Here's how the part is built. I have some questions about the finished solid (model axes, mm). A direction names the side the tool comes from. Round coordinates to 2 decimals unless told otherwise and drop trailing zeros. Order: outer loops, then holes, each group sorted by start corner. A loop starts at its lowest first (then second) coordinate and runs counter-clockwise, first axis right, second up. Notation, with made-up numbers: (52.25, 8) - (96.25, 8) arc R32 ccw to (96.25, 38) - close; hole circle Ø1 at (48, 32). An arc over 180 degrees is marked (long way). One line per item, written item: value.
from build123d import *
from OCP.BRepFilletAPI import BRepFilletAPI_MakeChamfer

# Parameters (mm, degrees)
SZKIC1_W                    = 50
SZKIC1_H                    = 20
DODANIE_WYCI_GNI_CIE1_DEPTH = 5
SZKIC2_W                    = 20
SZKIC2_H                    = 20
DODANIE_WYCI_GNI_CIE2_DEPTH = 20
SZKIC3_R                    = 2.5
WYTNIJ_WYCI_GNI_CIE1_DEPTH  = 60.371710435
ZAOKR_GLENIE1_R             = 10
SZKIC4_W                    = 50
SZKIC4_H                    = 5
DODANIE_WYCI_GNI_CIE3_DEPTH = 40
SFAZOWANIE1_SIZE            = 10
SFAZOWANIE1_SIZE2           = 37.320508076
SFAZOWANIE2_OUTLINE_R       = 2.5
SFAZOWANIE2_DEPTH           = 20
SFAZOWANIE2_START           = 30
SFAZOWANIE2_2_OUTLINE_R     = 2.5
SFAZOWANIE2_2_DEPTH         = 20
SZKIC5_R                    = 3.043345969
WYTNIJ_WYCI_GNI_CIE2_DEPTH  = 83.006097334


with BuildPart() as part:
    # Szkic1 → Dodanie-wyciągnięcie1 (new body)
    with BuildSketch(Plane.XY):
        with Locations((25, 10)):
            Rectangle(SZKIC1_W, SZKIC1_H)
    extrude(amount=DODANIE_WYCI_GNI_CIE1_DEPTH)

    # Szkic2 → Dodanie-wyciągnięcie2 (add)
    with BuildSketch(Plane.XY.offset(5)):
        with Locations((10, 10)):
            Rectangle(SZKIC2_W, SZKIC2_H)
        with Locations((40, 10)):
            Rectangle(SZKIC2_W, SZKIC2_H)
    extrude(amount=DODANIE_WYCI_GNI_CIE2_DEPTH)

    # Szkic3 → Wytnij-wyciągnięcie1 (cut, through all)
    with BuildSketch(Plane.ZY):
        with Locations((15, 10)):
            Circle(SZKIC3_R)
    extrude(amount=-WYTNIJ_WYCI_GNI_CIE1_DEPTH, mode=Mode.SUBTRACT)

    # Zaokrąglenie1
    zaokr_glenie1_edges = [part.edges().sort_by_distance(p)[0] for p in [
        (40, 20, 25),
        (40, 0, 25),
        (10, 0, 25),
        (10, 20, 25),
    ]]
    fillet(zaokr_glenie1_edges, radius=ZAOKR_GLENIE1_R - 0.0001)  # a hair under: the kernel refuses the full size

    # Szkic4 → Dodanie-wyciągnięcie3 (add)
    with BuildSketch(Plane(origin=(0, 20, 0), x_dir=(1, 0, 0), z_dir=(0, 1, 0))):
        with Locations((25, -2.5)):
            Rectangle(SZKIC4_W, SZKIC4_H)
    extrude(amount=DODANIE_WYCI_GNI_CIE3_DEPTH)

    # Sfazowanie1: one chamfer whose edges measure the first distance from different faces: ONE call of the kernel's chamfer builder (chamfer() names one face for all edges)
    sfazowanie1_edges_1 = [part.edges().sort_by_distance(p)[0] for p in [
        (40, 20, 5),
    ]]
    sfazowanie1_side_1 = [part.faces().sort_by_distance(p)[0] for p in [
        (40, 20, 10.00005),
    ]]
    sfazowanie1_edges_2 = [part.edges().sort_by_distance(p)[0] for p in [
        (10, 20, 5),
    ]]
    sfazowanie1_side_2 = [part.faces().sort_by_distance(p)[0] for p in [
        (10, 20, 10.00005),
    ]]
    sfazowanie1 = BRepFilletAPI_MakeChamfer(part.part.solid().wrapped)
    for e in sfazowanie1_edges_1:
        sfazowanie1.Add(SFAZOWANIE1_SIZE, SFAZOWANIE1_SIZE2, e.wrapped, sfazowanie1_side_1[0].wrapped)  # the first distance lies on this face
    for e in sfazowanie1_edges_2:
        sfazowanie1.Add(SFAZOWANIE1_SIZE, SFAZOWANIE1_SIZE2, e.wrapped, sfazowanie1_side_2[0].wrapped)  # the first distance lies on this face
    add(Compound.cast(sfazowanie1.Shape()), mode=Mode.REPLACE)

    # Sfazowanie2: read off the stored shape, not the designer's step
    # Sfazowanie2 outline → Sfazowanie2 (add)
    with BuildSketch(Plane.YZ):
        with BuildLine():
            Line((0, 15), (0, 0))
            Line((0, 0), (60, 0))
            Line((60, 0), (60, 5))
            Line((60, 5), (57.320508076, 5))
            Line((57.320508076, 5), (31.081570656, 12.030702092))
            Line((31.081570656, 12.030702092), (18.642014143, 20.031460181))
            ThreePointArc((18.642014143, 20.031460181), (7.394250725, 24.654536276), (0, 15))
        make_face()
        with Locations((10, 15)):
            Circle(SFAZOWANIE2_OUTLINE_R, mode=Mode.SUBTRACT)
    extrude(amount=SFAZOWANIE2_DEPTH)

    # Sfazowanie2 2 outline → Sfazowanie2 2 (add)
    with BuildSketch(Plane.YZ.offset(SFAZOWANIE2_START)):
        with BuildLine():
            Line((0, 15), (0, 0))
            Line((0, 0), (60, 0))
            Line((60, 0), (60, 5))
            Line((60, 5), (57.320508076, 5))
            Line((57.320508076, 5), (31.081570656, 12.030702092))
            Line((31.081570656, 12.030702092), (18.642014143, 20.031460181))
            ThreePointArc((18.642014143, 20.031460181), (7.394250725, 24.654536276), (0, 15))
        make_face()
        with Locations((10, 15)):
            Circle(SFAZOWANIE2_2_OUTLINE_R, mode=Mode.SUBTRACT)
    extrude(amount=SFAZOWANIE2_2_DEPTH)

    # Szkic5 → Wytnij-wyciągnięcie2 (cut, through all)
    with BuildSketch(Plane(origin=(0, 0, 0), x_dir=(-1, 0, 0), z_dir=(0, 0, -1))):
        with Locations((-42, 52)):
            Circle(SZKIC5_R)
        with Locations((-8, 52)):
            Circle(SZKIC5_R)
        with Locations((-8, 32)):
            Circle(SZKIC5_R)
        with Locations((-42, 32)):
            Circle(SZKIC5_R)
    extrude(amount=-WYTNIJ_WYCI_GNI_CIE2_DEPTH, mode=Mode.SUBTRACT)


solid = part.part
Q1. Will these pins go through, and if not, where does the flat tip stop? pin 1 (10 mm diameter, centred on x = 20.5, y = 38, fed in from +Z); pin 2 (3.5 mm diameter, centred on x = 8, y = 32, fed in from +Z); pin 3 (2 mm diameter, centred on x = 39, z = 14.5, fed in from +Y); pin 4 (9.5 mm diameter, centred on x = 42, y = 32, fed in from +Z).
Results list:
pin 1: z = 11.51
pin 2: through
pin 3: y = 28.8
pin 4: z = 14.5
Q2. We'd pull the mould along Z, two halves only. Please class faces 1 (the flat face through (9.86, 24.949, 15.975)), 2 (the flat face through (50, 23, 10)), 3 (the cylindrical face through (39.9, 8.5, 13)): released by +Z, released by -Z, zero draft, split by the parting line, or undercut.
Results list:
face 1: released by +Z
face 2: zero draft
face 3: undercut
Q3. If I drill on line 1 along X through (y, z) = (32, 7.5); line 2 along Y through (x, z) = (42, 2.5); line 3 along X through (y, z) = (17.5, 6), over which ranges is the centre line in solid material (lowest first)?
Results list:
line 1: 0 to 4.96, 11.04 to 20, 30 to 38.96, 45.04 to 50
line 2: 0 to 28.96, 35.04 to 48.96, 55.04 to 60
line 3: 0 to 20, 30 to 50
Q4. If we section it at D-D, the plane y = 4: Please give me the cut outline in (x, z), then the cut area to 3 significant figures.
Results list:
outline: (0, 0) - (50, 0) - (50, 23) - (30, 23) - (30, 5) - (20, 5) - (20, 23) - (0, 23) - close
area: 970 mm²
Q5. Which directions (+Z, -Z, +X, -X, +Y, -Y) give clear straight access to the entire face, cutting with the end or side of a thin tool? Please do faces 4 (the flat face through (30, 16, 13)), 5 (the flat face through (23, 34, 5)), 6 (the cylindrical face through (10.14, 3.01, 22.15)).
Results list:
face 4: +Z, +Y, -Y
face 5: +Z, +Y
face 6: +Z, +X, -X, -Y
Q6. If we section it at B-B, the plane z = 10.25: Please give me the cut outline in (x, y).
Results list:
outline: (0, 0) - (20, 0) - (20, 37.73) - (0, 37.73) - close; (30, 0) - (50, 0) - (50, 37.73) - (30, 37.73) - close; hole circle Ø6.09 at (8, 32); hole circle Ø6.09 at (42, 32)
Q7. If we section it at C-C, the plane y = 32: Please give me the cut outline in (x, z), then the cut area to 3 significant figures.
Results list:
outline: (0, 0) - (4.96, 0) - (4.96, 11.78) - (0, 11.78) - close; (11.04, 0) - (38.96, 0) - (38.96, 11.78) - (30, 11.78) - (30, 5) - (20, 5) - (20, 11.78) - (11.04, 11.78) - close; (45.04, 0) - (50, 0) - (50, 11.78) - (45.04, 11.78) - close
area: 378 mm²
